```python
from build123d import *

# Parameters (mm, degrees)
F0_W     = 889
F0_H     = 596.9
F1_DEPTH = 19.05
F3_R     = 12.7
F4_DEPTH = 25.4
F5_DEPTH = 25.4


with BuildPart() as f1:
    # F0 (on Top) → F1 (new body)
    with BuildSketch(Plane.XY):
        with Locations((444.5, 298.45)):
            Rectangle(F0_W, F0_H)
    extrude(amount=F1_DEPTH)

    # F3 (on face) → F4 (cut)
    with BuildSketch(Plane.XY.offset(19.05)):
        with Locations((38.1, 558.8)):
            Circle(F3_R)
        with Locations((139.7, 558.8)):
            Circle(F3_R)
        with Locations((241.3, 558.8)):
            Circle(F3_R)
        with Locations((342.9, 558.8)):
            Circle(F3_R)
        with Locations((444.5, 558.8)):
            Circle(F3_R)
        with Locations((546.1, 558.8)):
            Circle(F3_R)
        with Locations((647.7, 558.8)):
            Circle(F3_R)
        with Locations((749.3, 558.8)):
            Circle(F3_R)
        with Locations((850.9, 558.8)):
            Circle(F3_R)
        with Locations((342.9, 38.1)):
            Circle(F3_R)
        with Locations((850.9, 38.1)):
            Circle(F3_R)
        with Locations((139.7, 38.1)):
            Circle(F3_R)
        with Locations((241.3, 38.1)):
            Circle(F3_R)
        with Locations((647.7, 38.1)):
            Circle(F3_R)
        with Locations((749.3, 38.1)):
            Circle(F3_R)
        with Locations((38.1, 38.1)):
            Circle(F3_R)
        with Locations((444.5, 38.1)):
            Circle(F3_R)
        with Locations((546.1, 38.1)):
            Circle(F3_R)
        with Locations((38.1, 457.2)):
            Circle(F3_R)
        with Locations((38.1, 355.6)):
            Circle(F3_R)
        with Locations((38.1, 254)):
            Circle(F3_R)
        with Locations((38.1, 152.4)):
            Circle(F3_R)
        with Locations((850.9, 152.4)):
            Circle(F3_R)
        with Locations((850.9, 254)):
            Circle(F3_R)
        with Locations((850.9, 355.6)):
            Circle(F3_R)
        with Locations((850.9, 457.2)):
            Circle(F3_R)
    extrude(amount=-F4_DEPTH, mode=Mode.SUBTRACT)

    # F2 (on face) → F5 (cut)
    with BuildSketch(Plane.XY.offset(19.05)):
        with BuildLine():
            ThreePointArc((139.7, 463.55), (127, 450.85), (139.7, 438.15))
            Line((139.7, 438.15), (342.9, 438.15))
            ThreePointArc((342.9, 438.15), (355.6, 450.85), (342.9, 463.55))
            Line((342.9, 463.55), (139.7, 463.55))
        make_face()
        with BuildLine():
            ThreePointArc((749.3, 438.15), (762, 450.85), (749.3, 463.55))
            Line((749.3, 463.55), (546.1, 463.55))
            ThreePointArc((546.1, 463.55), (533.4, 450.85), (546.1, 438.15))
            Line((546.1, 438.15), (749.3, 438.15))
        make_face()
        with BuildLine():
            Line((342.9, 311.15), (139.7, 311.15))
            ThreePointArc((139.7, 311.15), (127, 298.45), (139.7, 285.75))
            Line((139.7, 285.75), (342.9, 285.75))
            ThreePointArc((342.9, 285.75), (355.6, 298.45), (342.9, 311.15))
        make_face()
        with BuildLine():
            Line((749.3, 311.15), (546.1, 311.15))
            ThreePointArc((546.1, 311.15), (533.4, 298.45), (546.1, 285.75))
            Line((546.1, 285.75), (749.3, 285.75))
            ThreePointArc((749.3, 285.75), (762, 298.45), (749.3, 311.15))
        make_face()
        with BuildLine():
            Line((139.7, 133.35), (342.9, 133.35))
            ThreePointArc((342.9, 133.35), (355.6, 146.05), (342.9, 158.75))
            Line((342.9, 158.75), (139.7, 158.75))
            ThreePointArc((139.7, 158.75), (127, 146.05), (139.7, 133.35))
        make_face()
        with BuildLine():
            ThreePointArc((546.1, 158.75), (533.4, 146.05), (546.1, 133.35))
            Line((546.1, 133.35), (749.3, 133.35))
            ThreePointArc((749.3, 133.35), (762, 146.05), (749.3, 158.75))
            Line((749.3, 158.75), (546.1, 158.75))
        make_face()
    extrude(amount=-F5_DEPTH, mode=Mode.SUBTRACT)


solid = f1.part
```
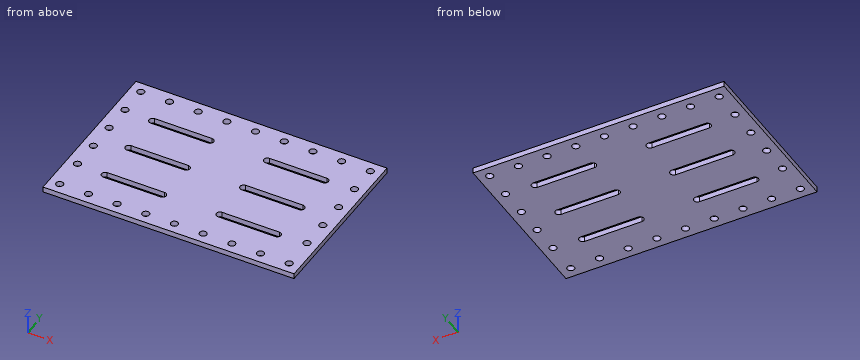
Could you check a few things on this model? Use its own coordinates, in mm. Round coordinates to 2 decimals unless told otherwise and drop trailing zeros. Loops run counter-clockwise (first coordinate to the right, second up) from the corner with the lowest first, then second, coordinate; pieces in that order, holes last. Notation, with made-up numbers: (46, 33) -> (72, 33) arc R12 cw to (72, 42) -> close; hole circle Ø1 at (-3, 44.5). An arc over 180 degrees is marked (long way). One line per question, with ' | ' between items.
(1) For pin 1 Ø23 at (x, y) = (38.1, 558.8) entering from +Z, with a flat end and sliding along its axis, tell me the tip position at first contact or that it passes through.
Model answer:
pin 1: passes through
(2) If we section it at A-A on x = 38.1: List the corners of the cut face in (y, z) for me, and give its area (3 significant figures).
Model answer:
outline: (0, 0) -> (25.4, 0) -> (25.4, 19.05) -> (0, 19.05) -> close; (50.8, 0) -> (139.7, 0) -> (139.7, 19.05) -> (50.8, 19.05) -> close; (165.1, 0) -> (241.3, 0) -> (241.3, 19.05) -> (165.1, 19.05) -> close; (266.7, 0) -> (342.9, 0) -> (342.9, 19.05) -> (266.7, 19.05) -> close; (368.3, 0) -> (444.5, 0) -> (444.5, 19.05) -> (368.3, 19.05) -> close; (469.9, 0) -> (546.1, 0) -> (546.1, 19.05) -> (469.9, 19.05) -> close; (571.5, 0) -> (596.9, 0) -> (596.9, 19.05) -> (571.5, 19.05) -> close | area: 8,470 mm^2
(3) If I drill on probe 1 along Y at (x, z) = (241.3, 4.75); probe 2 along Y at (x, z) = (620.5, 13.5), over which ranges is the centre line in solid material (lowest first)?
Model answer:
probe 1: y = 0 to 25.4, 50.8 to 133.35, 158.75 to 285.75, 311.15 to 438.15, 463.55 to 546.1, 571.5 to 596.9 | probe 2: y = 0 to 133.35, 158.75 to 285.75, 311.15 to 438.15, 463.55 to 596.9
(4) If we section it at B-B on y = 254: List the corners of the cut face in (x, z) for me.
Model answer:
outline: (0, 0) -> (25.4, 0) -> (25.4, 19.05) -> (0, 19.05) -> close; (50.8, 0) -> (838.2, 0) -> (838.2, 19.05) -> (50.8, 19.05) -> close; (863.6, 0) -> (889, 0) -> (889, 19.05) -> (863.6, 19.05) -> close
(5) If we section it at C-C on x = 584: List the corners of the cut face in (y, z) for me, and give its area (3 significant figures).
Model answer:
outline: (0, 0) -> (133.35, 0) -> (133.35, 19.05) -> (0, 19.05) -> close; (158.75, 0) -> (285.75, 0) -> (285.75, 19.05) -> (158.75, 19.05) -> close; (311.15, 0) -> (438.15, 0) -> (438.15, 19.05) -> (311.15, 19.05) -> close; (463.55, 0) -> (596.9, 0) -> (596.9, 19.05) -> (463.55, 19.05) -> close | area: 9,920 mm^2
(6) If we section it at D-D on y = 558.8: Count the separate pieces of the cut face and the enclosed holes in it, and give its area (3 significant figures).
Model answer:
separate pieces: 10 | enclosed holes: 0 | area: 12,600 mm^2
